Geometry check sheet. Reference: the model listing, model coordinates, mm. A direction names the side the tool comes from. Coordinates: 2 decimals unless noted, no trailing zeros. Order: outer loops, then holes, each group sorted by start corner. A loop starts at its lowest first (then second) coordinate and runs counter-clockwise, first axis right, second up. Notation, with made-up numbers: (38.25, 18) - (82.25, 18) arc R18 cw to (82.25, 45) - close; hole circle Ø8 at (41.5, -34). An arc over 180 degrees is marked (long way). One line per item, written item: value. Start each with the question number.
```python
from build123d import *

# Parameters (mm, degrees)
F0_W     = 82.55
F0_H     = 35.052
F1_DEPTH = 3.175
F3_D     = 3.81
F4_W     = 57.15
F4_H     = 35.052
F5_DEPTH = 31.75


with BuildPart() as f1:
    # F0 (on Top) → F1 (new body)
    with BuildSketch(Plane.XY):
        with Locations((1.768986, -20.037849)):
            Rectangle(F0_W, F0_H)
    extrude(amount=F1_DEPTH)

    # F3 (through all)
    with Locations(Plane.XY.offset(3.175)):
        with Locations((-34.443449, -8.69142)):
            Hole(F3_D / 2)

    # F4 (on Top) → F5 (join)
    with BuildSketch(Plane.XY):
        with Locations((1.768986, -20.037849)):
            Rectangle(F4_W, F4_H)
    extrude(amount=F5_DEPTH)


solid = f1.part
```
Q1. Gauge pin test, flat ends, axial feed: P1, Ø4, axis at x = -34.5, y = -16, coming from the +Z side (3 decimals); P2, Ø1, axis at y = -30, z = 22, coming from the +X side; P3, Ø2.5, axis at x = -34.44, y = -8.69, coming from the +Z side; P4, Ø1.5, axis at y = -29.5, z = 27, coming from the -X side. Record the tip position at first contact, or that the pin passes through.
Q2. Cross-section at A-A, the plane y = -12. Enter the section's corners in (x, z) (3 decimals).
Q3. Cross-section at C-C, the plane z = 14. Enter the section's corners in (x, y), and give its area (3 significant figures).
Q4. Material ranges on probe 1 along X at (y, z) = (-5, 12.5); probe 2 along Z at (x, y) = (-32, -11) (3 decimals), recorded low to high.
Q5. Release check for a two-part mould opening along X. For faces 4 (the cylindrical face through (-33.039, -7.404, 1.565)), 5 (the flat face through (1, -2.512, 16)), 6 (the flat face through (-26.806, -20, 17)), 7 (the flat face through (30.344, -20, 17)) record: released by +X, released by -X, zero draft, split by the parting line, or undercut.
Q6. Set-up check for faces 1 (the flat face through (-33, -20, 3.175)), 2 (the flat face through (37, -20, 3.175)), 3 (the flat face through (1, -37.564, 16)): record each of +Z, -Z, +X, -X, +Y, -Y from which the full face is reachable in a straight line by a thin tool's end or side.
Q7. Cross-section at B-B, the plane x = 34.5. Enter the section's corners in (y, z) (3 decimals), and give its area (3 significant figures).
Check result:
1. P1: stops at z = 3.175
1. P2: stops at x = 30.34
1. P3: passes through
1. P4: stops at x = -26.81
2. outline: (-39.506, 0) - (43.044, 0) - (43.044, 3.175) - (30.344, 3.175) - (30.344, 31.75) - (-26.806, 31.75) - (-26.806, 3.175) - (-39.506, 3.175) - close
3. outline: (-26.81, -37.56) - (30.34, -37.56) - (30.34, -2.51) - (-26.81, -2.51) - close
3. area: 2,000 mm2
4. probe 1: x = -26.81 to 30.34
4. probe 2: z = 0 to 3.175
5. face 4: undercut
5. face 5: zero draft
5. face 6: released by -X
5. face 7: released by +X
6. face 1: +Z, -X, +Y, -Y
6. face 2: +Z, +X, +Y, -Y
6. face 3: +Z, -Z, +X, -X, -Y
7. outline: (-37.564, 0) - (-2.512, 0) - (-2.512, 3.175) - (-37.564, 3.175) - close
7. area: 111 mm2
